Read the model definition and answer for the solid it produces. Units are mm, in the model's axes. Coordinates: 2 decimals unless noted, no trailing zeros. Write each loop counter-clockwise with the first axis right and the second up, starting at its lowest first coordinate (ties: lowest second). Pieces come first, ordered by that corner, then holes. Notation, with made-up numbers: (18, -14.75) -> (65, -14.75) arc R13 ccw to (65, 2.25) -> close; hole circle Ø4 at (65.25, 78.5). An arc over 180 degrees is marked (long way). Answer in a Markdown table with one row per item. Add a question column.
Item 1: Section C-C on y = 139 is taken. Write down the section's boundary in (x, z), then the cut area to 3 significant figures.
Item 2: Straight lines are drawn through the part: line 1 (Y direction, x = 0, z = -0.5); line 2 (X direction, y = -143, z = 0.5); line 3 (Y direction, x = 3.25, z = -0.75). For each, find the intervals that lie inside material, in ascending order. Write a range as from..to.
Item 3: For a pull along Y with two mould halves and no side action, classify faces 1 (the face through (-0.9, 2.45, -2.86)), 2 (the face through (-1, -175.35, 3)) as +Y half, -Y half, draft (parallel to the pull), parting line (faces both ways), or undercut.
Item 4: Section B-B on x = 0 is taken. Write down the section's boundary in (y, z).
Item 5: Given pin 1 Ø2 at (x, y) = (1.5, 60.5) entering from +Z; pin 2 Ø6 at (y, z) = (-102, -2.5) entering from +X; pin 3 Ø3.5 at (x, z) = (1.5, -1.5) entering from -Y; pin 4 Ø4.5 at (x, z) = (0.5, -1) entering from +Y, each flat-ended and moving along its own axis, determine where each tip first touches the part or whether it passes through.
Item 6: Section A-A on z = 0 is taken. Write down the section's boundary in (x, y).
```python
from build123d import *

# Parameters (mm, degrees)
SKETCH_1_W = 1
SKETCH_1_H = 350.7


with BuildPart() as part:
    # Эскиз1 → Повернуть1 (revolve)
    with BuildSketch(Plane.XY, mode=Mode.PRIVATE) as revolve_1_sk:
        with Locations((2.5, 0)):
            Rectangle(SKETCH_1_W, SKETCH_1_H)
    revolve(revolve_1_sk.sketch.rotate(Axis((0, 0, 0), (0, 1, 0)), 90), axis=Axis((0, 0, 0), (0, 1, 0)))

    # Эскиз2 → Повернуть5 (revolve)
    with BuildSketch(Plane.XY):
        with BuildLine():
            Line((0, 175.35), (0, 186.35))
            ThreePointArc((0, 186.35), (5.744562647, 182.082050808), (3.31662479, 175.35))
            Line((3.31662479, 175.35), (0, 175.35))
        make_face()
    revolve_5 = revolve(axis=Axis((0, 175.35, 0), (0, 1, 0)))

    # Зеркальное отражение1: Повернуть5 across plane
    add(revolve_5.mirror(Plane.ZX))


solid = part.part
```
Results below:
| question | item | result |
|---|---|---|
| 1 | outline | circle Ø6 at (0, 0); hole circle Ø4 at (0, 0) |
| 1 | area | 15.7 mm2 |
| 2 | line 1 | y = -186.33..-175.35, 175.35..186.33 |
| 2 | line 2 | x = -2.96..-1.94, 1.94..2.96 |
| 2 | line 3 | y = -185.34..-175.36, 175.36..185.34 |
| 3 | face 1 | undercut |
| 3 | face 2 | undercut |
| 4 | outline | (-175.35, -3.32) -> (-175.35, -3) -> (175.35, -3) -> (175.35, -3.32) arc R6 ccw (long way) to (175.35, 3.32) -> (175.35, 3) -> (-175.35, 3) -> (-175.35, 3.32) arc R6 ccw (long way) to start; hole (-175.35, -2) -> (175.35, -2) -> (175.35, 2) -> (-175.35, 2) -> close |
| 5 | pin 1 | stops at z = 2.96 |
| 5 | pin 2 | stops at x = 3 |
| 5 | pin 3 | stops at y = -186.34 |
| 5 | pin 4 | stops at y = 186.35 |
| 6 | outline | (-3.32, -175.35) arc R6 ccw (long way) to (3.32, -175.35) -> (3, -175.35) -> (3, 175.35) -> (3.32, 175.35) arc R6 ccw (long way) to (-3.32, 175.35) -> (-3, 175.35) -> (-3, -175.35) -> close; hole (-2, -175.35) -> (2, -175.35) -> (2, 175.35) -> (-2, 175.35) -> close |
